from build123d import *

# Parameters (mm, degrees)
SKETCH1_W           = 368.3
SKETCH1_H           = 111.125
BOSS_EXTRUDE1_DEPTH = 101.6
SKETCH2_R           = 114.3
BOSS_EXTRUDE2_DEPTH = 19.05
SKETCH3_R           = 87.63
BOSS_EXTRUDE3_DEPTH = 12.7
SKETCH4_R           = 12.5
BOSS_EXTRUDE4_DEPTH = 69.85
SKETCH5_W           = 355.6
SKETCH5_H           = 304.8
BOSS_EXTRUDE5_DEPTH = 101.6
SKETCH6_R           = 92.075
BOSS_EXTRUDE6_DEPTH = 3.175
DOME1_FACE_RADIUS   = 92.075
DOME1_HEIGHT        = 17.78
FILLET1_R           = 15.24
SKETCH7_W           = 152.4
SKETCH7_H           = 101.6
BOSS_EXTRUDE7_DEPTH = 76.2
SKETCH8_R           = 12.660326574
SKETCH8_R_2         = 10.120326574
EXTRUDE_THIN1_DEPTH = 25.4
CUT_EXTRUDE1_REACH  = 245.205
SKETCH9_R           = 4.365625


with BuildPart() as part:
    # Sketch1 → Boss-Extrude1 (new body)
    with BuildSketch(Plane(origin=(0, 0, 0), x_dir=(1, 0, 0), z_dir=(0, 1, 0))):
        with Locations((-63.5, 0)):
            Rectangle(SKETCH1_W, SKETCH1_H)
    extrude(amount=BOSS_EXTRUDE1_DEPTH)

    # Sketch2 → Boss-Extrude2 (add)
    with BuildSketch(Plane.XZ):
        with Locations(Location((0, 0, 0), (0, 0, 29.085295061))):  # turned: the seam where the file's is
            Circle(SKETCH2_R)
    extrude(amount=BOSS_EXTRUDE2_DEPTH)

    # Sketch3 → Boss-Extrude3 (add)
    with BuildSketch(Plane.XZ.offset(19.05)):
        with Locations(Location((0, 0, 0), (0, 0, 270))):  # turned: the seam where the file's is
            Circle(SKETCH3_R)
    extrude(amount=BOSS_EXTRUDE3_DEPTH)

    # Sketch4 → Boss-Extrude4 (add)
    with BuildSketch(Plane.XZ.offset(31.75)):
        with Locations(Location((0, 0, 0), (0, 0, 270))):  # turned: the seam where the file's is
            Circle(SKETCH4_R)
    extrude(amount=BOSS_EXTRUDE4_DEPTH)

    # Sketch5 → Boss-Extrude5 (add)
    with BuildSketch(Plane(origin=(0, 101.6, 0), x_dir=(1, 0, 0), z_dir=(0, 1, 0))):
        with Locations((-19.05, 0)):
            Rectangle(SKETCH5_W, SKETCH5_H)
    extrude(amount=BOSS_EXTRUDE5_DEPTH)

    # Sketch6 → Boss-Extrude6 (add)
    with BuildSketch(Plane(origin=(0, 203.2, 0), x_dir=(1, 0, 0), z_dir=(0, 1, 0))):
        with Locations(Location((0, 0, 0), (0, 0, 90))):  # turned: the seam where the file's is
            Circle(SKETCH6_R)
    extrude(amount=BOSS_EXTRUDE6_DEPTH)

    # Dome1: a dome of height H over a round flat face of radius A is a cap of a sphere of radius (A * A + H * H) / (2 * H)
    dome1_r = (DOME1_FACE_RADIUS * DOME1_FACE_RADIUS + DOME1_HEIGHT * DOME1_HEIGHT) / (2 * DOME1_HEIGHT)
    dome1_base = Plane((0, 206.375, 0), z_dir=(0, 1, 0))
    with Locations(dome1_base.offset(DOME1_HEIGHT - dome1_r)):
        dome1_ball = Sphere(dome1_r, mode=Mode.PRIVATE)
    add(split(dome1_ball, bisect_by=dome1_base, keep=Keep.TOP, mode=Mode.PRIVATE))

    # Fillet1
    fillet1_edges = [part.edges().sort_by_distance(p)[0] for p in [
        (158.75, 152.4, 152.4),
        (158.75, 152.4, -152.4),
        (-196.85, 152.4, -152.4),
        (-196.85, 152.4, 152.4),
    ]]
    fillet(fillet1_edges, radius=FILLET1_R)

    # Sketch7 → Boss-Extrude7 (add)
    with BuildSketch(Plane.XY.offset(55.5625)):
        with Locations((-171.45, 50.8)):
            Rectangle(SKETCH7_W, SKETCH7_H)
    extrude(amount=BOSS_EXTRUDE7_DEPTH)

    # Sketch8 → Extrude-Thin1 (add)
    with BuildSketch(Plane.ZY.offset(247.65)):
        with Locations((115.540395057, 68.867744931)):
            Circle(SKETCH8_R)
        with Locations((115.540395057, 68.867744931)):
            Circle(SKETCH8_R_2, mode=Mode.SUBTRACT)
    extrude(amount=EXTRUDE_THIN1_DEPTH)

    # Sketch9 → Cut-Extrude1 (cut, up to next)
    with BuildSketch(Plane.XZ.offset(19.05), mode=Mode.PRIVATE) as cut_extrude1_sk1:
        with Locations(Location((39.624, 93.472, 0), (0, 0, 270))):  # turned: the seam where the file's is
            Circle(SKETCH9_R)
    cut_extrude1_tool1 = extrude(cut_extrude1_sk1.sketch, amount=-CUT_EXTRUDE1_REACH, mode=Mode.PRIVATE) & part.part
    add(cut_extrude1_tool1.solids().sort_by_distance((39.624, -19.05, 93.472))[0], mode=Mode.SUBTRACT)
    # Sketch9 → Cut-Extrude1 (cut, up to next)
    with BuildSketch(Plane.XZ.offset(19.05), mode=Mode.PRIVATE) as cut_extrude1_sk2:
        with Locations(Location((76.708, -66.548, 0), (0, 0, 270))):  # turned: the seam where the file's is
            Circle(SKETCH9_R)
    cut_extrude1_tool2 = extrude(cut_extrude1_sk2.sketch, amount=-CUT_EXTRUDE1_REACH, mode=Mode.PRIVATE) & part.part
    add(cut_extrude1_tool2.solids().sort_by_distance((76.708, -19.05, -66.548))[0], mode=Mode.SUBTRACT)
    # Sketch9 → Cut-Extrude1 (cut, up to next)
    with BuildSketch(Plane.XZ.offset(19.05), mode=Mode.PRIVATE) as cut_extrude1_sk3:
        with Locations(Location((-81.28, -61.214, 0), (0, 0, 270))):  # turned: the seam where the file's is
            Circle(SKETCH9_R)
    cut_extrude1_tool3 = extrude(cut_extrude1_sk3.sketch, amount=-CUT_EXTRUDE1_REACH, mode=Mode.PRIVATE) & part.part
    add(cut_extrude1_tool3.solids().sort_by_distance((-81.28, -19.05, -61.214))[0], mode=Mode.SUBTRACT)


solid = part.part
The listing builds one solid part. Answer for the finished solid, in the listing's coordinates (mm). A direction names the side the tool comes from. Coordinates: 2 decimals unless noted, no trailing zeros. Loops run counter-clockwise (first coordinate to the right, second up) from the corner with the lowest first, then second, coordinate; pieces in that order, holes last.
1) Find section B-B on z = 0. Write down the section's boundary in (x, y) (3 decimals).
2) Determine the mould class of faces 5 (the face through (-260.172, 71.908, 125.193)), 6 (the face through (3.755, -66.186, -11.923)), 7 (the face through (-192.5, 153.11, -147.82)) for opening direction Z: pulls with the +Z half, pulls with the -Z half, needs draft (parallel to the pull), parting line crosses it, or undercut.
3) Flat-ended cylindrical pins translate along their axes: pin 1 Ø1.5 at (y, z) = (-55.5, -5) entering from -X; pin 2 Ø23 at (x, z) = (111.5, -8.5) entering from -Y; pin 3 Ø10 at (y, z) = (68, 114) entering from -X. Find the tip coordinate at first contact, or state that the pin passes through.
4) Find section D-D on y = 173.5. Write down the section's boundary in (x, z), then the cut area to 3 significant figures.
5) Find section A-A on z = -101. Write down the section's boundary in (x, y).
6) A tool of negligible diameter and unlimited length cuts with its end or side. For faces 1 (the face through (-260.172, 72.671, 127.616)), 2 (the face through (-223, 101.6, 37)), 3 (the face through (32.588, -9.392, -109.556)), 4 (the face through (-101, 203.2, -2)), from which of +Z, -Z, +X, -X, +Y, -Y can it reach the whole face along a straight path? Write none if from no direction.
7) Find the intervals of material crossed by L1, parallel to Y at x = -61, z = -80; L2, parallel to Y at x = -198.5, z = -14; L3, parallel to Y at x = -96.5, z = -139, in increasing order.
Values:
1. outline: (-247.65, 0) - (-114.3, 0) - (-114.3, -19.05) - (-87.63, -19.05) - (-87.63, -31.75) - (-12.5, -31.75) - (-12.5, -101.6) - (12.5, -101.6) - (12.5, -31.75) - (87.63, -31.75) - (87.63, -19.05) - (114.3, -19.05) - (114.3, 0) - (120.65, 0) - (120.65, 101.6) - (158.75, 101.6) - (158.75, 203.2) - (92.075, 203.2) - (92.075, 206.375) arc R247.298 ccw to (-92.075, 206.375) - (-92.075, 203.2) - (-196.85, 203.2) - (-196.85, 101.6) - (-247.65, 101.6) - close
2. face 5: undercut
2. face 6: parting line crosses it
2. face 7: pulls with the -Z half
3. pin 1: stops at x = -11.76
3. pin 2: stops at y = -19.05
3. pin 3: stops at x = -247.65
4. outline: (-196.85, -137.16) arc R15.24 ccw to (-181.61, -152.4) - (143.51, -152.4) arc R15.24 ccw to (158.75, -137.16) - (158.75, 137.16) arc R15.24 ccw to (143.51, 152.4) - (-181.61, 152.4) arc R15.24 ccw to (-196.85, 137.16) - close
4. area: 108,000 mm2
5. outline: (-196.85, 101.6) - (158.75, 101.6) - (158.75, 203.2) - (-196.85, 203.2) - close; (-53.51, -19.05) - (53.51, -19.05) - (53.51, 0) - (-53.51, 0) - close
6. face 1: -X
6. face 2: +Z, -Z, -X, +Y
6. face 3: -Y
6. face 4: +Y
7. L1: y = -19.05 to 0, 101.6 to 203.2
7. L2: y = 0 to 101.6
7. L3: y = 101.6 to 203.2
